Part model, mm, in its own coordinate system. Give positions to 0.01 mm unless a question says otherwise; leave off trailing zeros. Write each loop counter-clockwise with the first axis right and the second up, starting at its lowest first coordinate (ties: lowest second). Pieces come first, ordered by that corner, then holes.
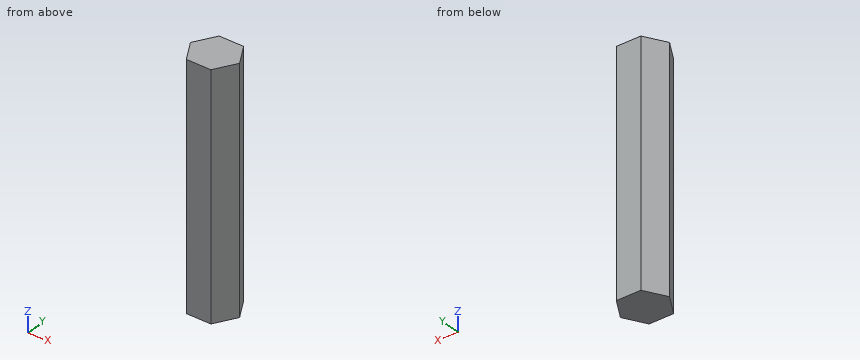
from build123d import *


with BuildPart() as f2:
    # F2: sweep along a path in F1
    with BuildLine(Plane.YZ) as f2_path:
        Line((0, 0), (0, 107.95))
    # F0 (on Top) → F2 (sweep)
    with BuildSketch(Plane.XY):
        Polygon((5.520493, -9.51271), (10.998495, 0.024532), (5.478003, 9.537242), (-5.520493, 9.51271), (-10.998495, -0.024532), (-5.478003, -9.537242), align=None)
    sweep(path=f2_path.line)


solid = f2.part
1) Saw through at B-B (x = -7.25). Write the cut outline in (y, z), and give its area (3 significant figures).
Check result:
outline: (-6.48, 0) - (6.5, 0) - (6.5, 107.95) - (-6.48, 107.95) - close
area: 1,400 mm2
2) Drill centre lines: L1, parallel to Y at x = -3.25, z = 65; L2, parallel to X at y = 0, z = 83.5; L3, parallel to X at y = 5, z = 65.5. Where is each one in solid material? Low to high.
Check result:
L1: y = -9.53 to 9.52
L2: x = -10.98 to 10.98
L3: x = -8.11 to 8.11
3) Saw through at A-A (z = 31). Write the cut outline in (x, y), and give its area (3 significant figures).
Check result:
outline: (-11, -0.02) - (-5.48, -9.54) - (5.52, -9.51) - (11, 0.02) - (5.48, 9.54) - (-5.52, 9.51) - close
area: 314 mm2
4) Saw through at C-C (y = -3.25). Write the cut outline in (x, z), and give its area (3 significant figures).
Check result:
outline: (-9.13, 0) - (9.12, 0) - (9.12, 107.95) - (-9.13, 107.95) - close
area: 1,970 mm2
5) Flat gauge pins, fed straight in: P1, Ø4, axis at y = -2.5, z = 50, coming from the -X side; P2, Ø6, axis at y = -6, z = 94, coming from the +X side; P3, Ø3, axis at y = -1.5, z = 30.5, coming from the +X side. Where does each tip first touch, or does it go through?
Check result:
P1: stops at x = -10.72
P2: stops at x = 9.26
P3: stops at x = 10.98
